Design review of the part built by this model. Coordinates are the model's own, in mm. Face numbers are marked on the shaded views. A direction names the side the tool comes from. Give positions to 0.01 mm unless a question says otherwise; leave off trailing zeros. Loops run counter-clockwise (first coordinate to the right, second up) from the corner with the lowest first, then second, coordinate; pieces in that order, holes last. Notation, with made-up numbers: (85, 44.25) - (119, 44.25) arc R22 cw to (119, 64.25) - close; hole circle Ø10 at (59.5, 13.5). An arc over 180 degrees is marked (long way). Put each result on its own line as item: value. Start each with the question number.
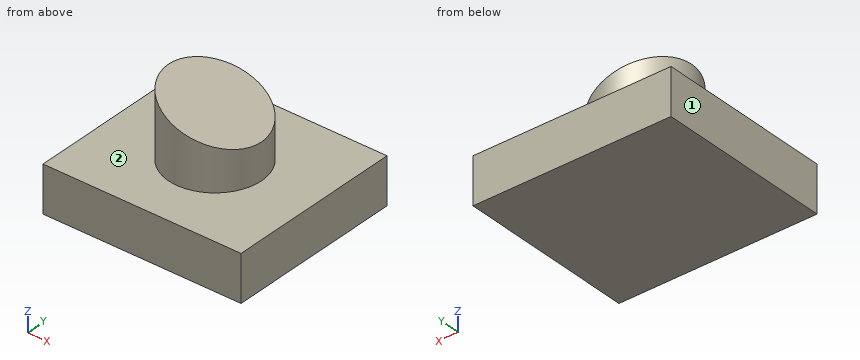
```python
from build123d import *

# Parameters (mm, degrees)
F0_W     = 108.696282
F0_H     = 97.515046
F1_DEPTH = 25.4
F2_R     = 25.511532
F3_DEPTH = 38.1
F5_DEPTH = 63.5


with BuildPart() as f1:
    # F0 (on Top) → F1 (new body)
    with BuildSketch(Plane.XY):
        Rectangle(F0_W, F0_H)
    extrude(amount=-F1_DEPTH)

    # F2 (on Top) → F3 (join)
    with BuildSketch(Plane.XY):
        Circle(F2_R)
    extrude(amount=F3_DEPTH)

    # F4 (on Front) → F5 (cut, symmetric)
    with BuildSketch(Plane.XZ):
        Polygon((25.862852, 41.473117), (-35.257578, 41.473117), (25.597604, 19.722745), align=None)
    extrude(amount=F5_DEPTH, both=True, mode=Mode.SUBTRACT)


solid = f1.part
```
Item 1: Consider section C-C (z = 8.5). State the section outline as (x, y) points.
Item 2: For L1, parallel to Z at x = 47, y = -20; L2, parallel to X at y = 0, z = 16.5; L3, parallel to Z at x = 0.5, y = -9, list the stretches that pass through material, from the lowest coordinate up. Write a range as from..to.
Item 3: Consider section A-A (y = 0). State the section outline as (x, z) points, plus the area to 3 significant figures.
Item 4: For P1, Ø2, axis at x = -29, y = 16, coming from the +Z side; P2, Ø6, axis at x = 0, z = 9.5, coming from the -Y side; P3, Ø1.5, axis at y = -11.5, z = 23.5, coming from the -X side, all flat-tipped, find the tip position at first contact; note any pin that passes through.
Item 5: Machinability: for the marked faces 1 and 2, which of the approach directions +Z, -Z, +X, -X, +Y, -Y give a long, thin tool a straight path to every point of the face, cutting with its end or side? Answer none if there is none.
Item 6: Consider section B-B (x = -10). State the section outline as (y, z) points, plus the area to 3 significant figures.
Item 7: Consider section D-D (x = 30). State the section outline as (y, z) points.
Geometry says:
1. outline: circle Ø51.02 at (0, 0)
2. L1: z = -25.4..0
2. L2: x = -25.51..25.51
2. L3: z = -25.4..28.69
3. outline: (-54.35, -25.4) - (54.35, -25.4) - (54.35, 0) - (25.51, 0) - (25.51, 19.75) - (-25.51, 37.99) - (-25.51, 0) - (-54.35, 0) - close
3. area: 4,230 mm2
4. P1: stops at z = 0
4. P2: stops at y = -25.51
4. P3: stops at x = -23.14
5. face 1: +Z, -Z, -X, +Y, -Y
5. face 2: +Z
6. outline: (-48.76, -25.4) - (48.76, -25.4) - (48.76, 0) - (23.47, 0) - (23.47, 32.45) - (-23.47, 32.45) - (-23.47, 0) - (-48.76, 0) - close
6. area: 4,000 mm2
7. outline: (-48.76, -25.4) - (48.76, -25.4) - (48.76, 0) - (-48.76, 0) - close
